```python
from build123d import *

# Parameters (mm, degrees)
PAD004_DEPTH    = 8.2
SKETCH014_W     = 28.5
SKETCH014_H     = 6.2
PAD005_DEPTH    = 1.8
SKETCH015_R     = 2.9
POCKET004_DEPTH = 0.6
SKETCH016_W     = 2.05
SKETCH016_H     = 6.2
POCKET005_DEPTH = 1.8
POCKET006_DEPTH = 4
SKETCH019_R     = 2.55
POCKET008_DEPTH = 7.5
SKETCH020_R     = 7
POCKET_DEPTH    = 3


with BuildPart() as part:
    # Sketch013 → Pad004 (new body)
    with BuildSketch(Plane.XY):
        with BuildLine():
            Line((0, 0), (28.5, 0))
            Line((28.5, 0), (28.5, 22.75))
            Line((28.5, 22.75), (14, 22.75))
            Line((14, 22.75), (14, 22.5))
            ThreePointArc((11, 19.5), (13.12132, 20.37868), (14, 22.5))
            Line((11, 19.5), (0, 19.5))
            Line((0, 19.5), (0, 0))
        make_face()
    extrude(amount=PAD004_DEPTH)

    # Sketch014 (on Face9 of Pad004) → Pad005 (join)
    with BuildSketch(Plane.XY.offset(8.2)):
        with Locations((14.25, 9.75)):
            Rectangle(SKETCH014_W, SKETCH014_H)
    extrude(amount=PAD005_DEPTH)

    # Sketch015 (on Face11 of Pad005) → Pocket004 (cut)
    with BuildSketch(Plane.XY.offset(10)):
        with Locations((8.735056, 9.75)):
            Circle(SKETCH015_R)
    extrude(amount=-POCKET004_DEPTH, mode=Mode.SUBTRACT)

    # Sketch016 (on Face10 of Pocket004) → Pocket005 (cut)
    with BuildSketch(Plane.XY.offset(10)):
        with Locations((15.5, 9.75)):
            Rectangle(SKETCH016_W, SKETCH016_H)
        Polygon((21.525, 12.85), (21.525, 6.65), (19.475, 6.65), (19.475, 12.85), (20.5, 12.85), align=None)
        with Locations((25.5, 9.75)):
            Rectangle(SKETCH016_W, SKETCH016_H)
    extrude(amount=-POCKET005_DEPTH, mode=Mode.SUBTRACT)

    # Sketch017 (on Face19 of Clone) → Pocket006 (cut)
    with BuildSketch(Plane.XY.offset(8.2)):
        with BuildLine():
            Line((0, 5.65), (13.475, 5.65))
            ThreePointArc((13.475, 5.65), (14.182107, 5.942893), (14.475, 6.65))
            Line((14.475, 6.65), (14.475, 16.75))
            Line((14.475, 16.75), (16.525, 16.75))
            Line((16.525, 16.75), (16.525, 5.65))
            Line((16.525, 5.65), (18.475, 5.65))
            ThreePointArc((18.475, 5.65), (19.182107, 5.942893), (19.475, 6.65))
            Line((19.475, 6.65), (19.475, 16.75))
            Line((19.475, 16.75), (21.525, 16.75))
            Line((21.525, 16.75), (21.525, 5.649972))
            Line((21.525, 5.649972), (23.475, 5.649972))
            ThreePointArc((23.475, 5.649972), (24.182107, 5.942865), (24.475, 6.649972))
            Line((24.475, 6.649972), (24.475, 16.75))
            Line((24.475, 16.75), (26.525, 16.75))
            Line((26.525, 16.75), (26.525, 5.65))
            ThreePointArc((24.475, 3.6), (25.924569, 4.200431), (26.525, 5.65))
            Line((24.475, 3.6), (0, 3.6))
            Line((0, 3.6), (0, 5.65))
        make_face()
    extrude(amount=-POCKET006_DEPTH, mode=Mode.SUBTRACT)

    # Sketch019 (on Face37 of Pocket006) → Pocket008 (cut)
    with BuildSketch(Plane.XY.offset(9.4)):
        with Locations((8.735056, 9.75)):
            Circle(SKETCH019_R)
    extrude(amount=-POCKET008_DEPTH, mode=Mode.SUBTRACT)

    # Sketch020 (on Face4 of Pocket008) → Pocket (cut)
    with BuildSketch(Plane(origin=(0, 0, 0), x_dir=(1, 0, 0), z_dir=(0, 0, -1))):
        with Locations((8.735056, -9.75)):
            Circle(SKETCH020_R)
    extrude(amount=-POCKET_DEPTH, mode=Mode.SUBTRACT)


solid = part.part
```
Here's how the part is built. I have some questions about the finished solid (model axes, mm). A direction names the side the tool comes from. Give positions to 0.01 mm unless a question says otherwise; leave off trailing zeros. Order: outer loops, then holes, each group sorted by start corner. A loop starts at its lowest first (then second) coordinate and runs counter-clockwise, first axis right, second up. Notation, with made-up numbers: (-6.5, 36.25) - (7.5, 36.25) arc R28 ccw to (7.5, 68.25) - close; hole circle Ø10 at (38.5, 1.5). An arc over 180 degrees is marked (long way). Answer as a JSON object with one key per item and string values. Group by question number.
Item 1: If we section it at A-A on z = 5.75: Please give me the cut outline in (x, y) (3 decimals), and give its area (3 significant figures).
Item 2: If we section it at D-D on y = 16.25: Please give me the cut outline in (x, z) (3 decimals), and give its area (3 significant figures).
Item 3: If we section it at C-C on x = 9: Please give me the cut outline in (y, z), and give its area (3 significant figures).
Item 4: Which directions (+Z, -Z, +X, -X, +Y, -Y) give clear straight access to the entire face, cutting with the end or side of a thin tool? Please do faces 1 (the flat face through (14, 2, 8.2)), 2 (the flat face through (9, 13, 3)), 3 (the flat face through (0, 10, 4)), 4 (the flat face through (24.475, 12, 7)), 5 (the flat face through (18, 12.85, 9)).
Item 5: For P1, Ø0.9, axis at x = 17.5, z = 9, coming from the +Y side; P2, Ø1.5, axis at x = 7.5, y = 12, coming from the -Z side; P3, Ø5, axis at x = 8.74, y = 9.75, coming from the -Z side; P4, Ø2, axis at x = 12.5, y = 17, coming from the +Z side, each with a flat end and sliding along its axis, tell me the tip position at first contact or that it passes through.
Item 6: If we mould it in two halves opening along X, with no side actions, what happens to faces 6 (the cylindrical face through (19.174, 5.935, 6.228)), 7 (the flat face through (23, 6, 8.2)), 8 (the cylindrical face through (13.1, 20.36, 4.04))? For each: pulls with the +X half, pulls with the -X half, needs draft (parallel to the pull), parting line crosses it, or undercut.
Item 7: If we section it at B-B on y = 9.75: Please give me the cut outline in (x, z) (3 decimals), and give its area (3 significant figures).
Item 8: Please list where these lines run through material, in increasing order: probe 1 along X at (y, z) = (9.75, 2.3); probe 2 along Y at (x, z) = (4, 7.25); probe 3 along Y at (x, z) = (21.75, 8).
Result set:
{
 "1": {"outline": "(0, 0) - (28.5, 0) - (28.5, 22.75) - (14, 22.75) - (14, 22.5) arc R3 cw to (11, 19.5) - (0, 19.5) - (0, 5.65) - (13.475, 5.65) arc R1 ccw to (14.475, 6.65) - (14.475, 16.75) - (16.525, 16.75) - (16.525, 5.65) - (18.475, 5.65) arc R1 ccw to (19.475, 6.65) - (19.475, 16.75) - (21.525, 16.75) - (21.525, 5.65) - (23.475, 5.65) arc R1 ccw to (24.475, 6.65) - (24.475, 16.75) - (26.525, 16.75) - (26.525, 5.65) arc R2.05 cw to (24.475, 3.6) - (0, 3.6) - close; hole circle Ø5.1 at (8.735, 9.75)", "area": "462 mm²"},
 "2": {"outline": "(0, 0) - (6.137, 0) - (6.137, 3) - (11.333, 3) - (11.333, 0) - (28.5, 0) - (28.5, 8.2) - (26.525, 8.2) - (26.525, 4.2) - (24.475, 4.2) - (24.475, 8.2) - (21.525, 8.2) - (21.525, 4.2) - (19.475, 4.2) - (19.475, 8.2) - (16.525, 8.2) - (16.525, 4.2) - (14.475, 4.2) - (14.475, 8.2) - (0, 8.2) - close", "area": "194 mm²"},
 "3": {"outline": "(0, 0) - (2.76, 0) - (2.76, 3) - (7.21, 3) - (7.21, 9.4) - (6.86, 9.4) - (6.86, 10) - (6.65, 10) - (6.65, 8.2) - (5.65, 8.2) - (5.65, 4.2) - (3.6, 4.2) - (3.6, 8.2) - (0, 8.2) - close; (12.29, 3) - (16.74, 3) - (16.74, 0) - (19.5, 0) - (19.5, 8.2) - (12.85, 8.2) - (12.85, 10) - (12.64, 10) - (12.64, 9.4) - (12.29, 9.4) - close", "area": "85.0 mm²"},
 "4": {"face 1": "+Z, +X, -X, -Y", "face 2": "-Z", "face 3": "+Z, -Z, -X, +Y, -Y", "face 4": "+Z", "face 5": "+Z, +X, -X, +Y"},
 "5": {"P1": "y = 12.85", "P2": "z = 3", "P3": "through", "P4": "z = 8.2"},
 "6": {"face 6": "undercut", "face 7": "needs draft", "face 8": "pulls with the -X half"},
 "7": {"outline": "(0, 0) - (1.735, 0) - (1.735, 3) - (6.185, 3) - (6.185, 9.4) - (5.835, 9.4) - (5.835, 10) - (0, 10) - close; (11.285, 3) - (15.735, 3) - (15.735, 0) - (28.5, 0) - (28.5, 10) - (26.525, 10) - (26.525, 4.2) - (24.475, 4.2) - (24.475, 10) - (21.525, 10) - (21.525, 4.2) - (19.475, 4.2) - (19.475, 10) - (16.525, 10) - (16.525, 4.2) - (14.475, 4.2) - (14.475, 10) - (11.635, 10) - (11.635, 9.4) - (11.285, 9.4) - close", "area": "171 mm²"},
 "8": {"probe 1": "0 to 1.74, 15.74 to 28.5", "probe 2": "0 to 3.6, 5.65 to 19.5", "probe 3": "0 to 3.6, 5.65 to 22.75"}
}
